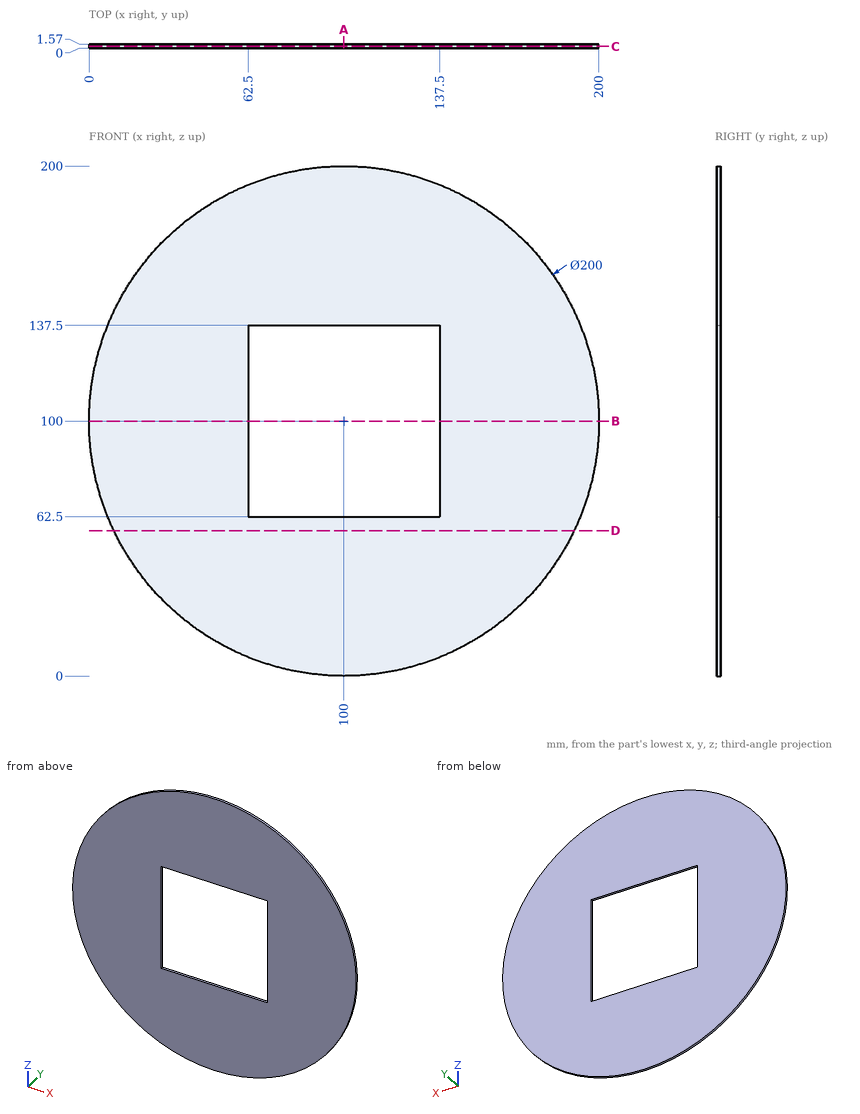
Here's the drawing with two shaded views (mm, measured from the low corner). I have some questions. Give positions to 0.01 mm unless a question says otherwise; leave off trailing zeros. Loops run counter-clockwise (first coordinate to the right, second up) from the corner with the lowest first, then second, coordinate; pieces in that order, holes last. Notation, with made-up numbers: (-14, 69) - (25, 69) arc R32 cw to (25, 97) - close; hole circle Ø7 at (62.25, 63). An arc over 180 degrees is marked (long way). Answer in a Markdown table with one row per item. Add a question column.
Q1. Please list where these lines run through material, in increasing order: L1, parallel to X at y = 0.9, z = 108; L2, parallel to X at y = 1, z = 130; L3, parallel to Z at x = 86.5, y = 0.85. Write a range as from..to.
Q2. If we section it at D-D (z = 57): List the corners of the cut face in (x, y) for me.
Q3. If we section it at B-B (z = 100): List the corners of the cut face in (x, y) for me, plus the area to 3 significant figures.
Q4. If we section it at A-A (x = 100): List the corners of the cut face in (y, z) for me.
Q5. For pin 1 (0.5 mm diameter, centred on y = 0.5, z = 88, fed in from +X); pin 2 (0.8 mm diameter, centred on x = 92, y = 1, fed in from -Z), each with a flat end and sliding along its axis, tell me the tip position at first contact or that it passes through.
Q6. If we section it at C-C (y = 0.6): List the corners of the cut face in (x, z) for me.
The answers:
| question | item | result |
|---|---|---|
| 1 | L1 | x = 0.32..62.5, 137.5..199.68 |
| 1 | L2 | x = 4.61..62.5, 137.5..195.39 |
| 1 | L3 | z = 0.92..62.5, 137.5..199.08 |
| 2 | outline | (9.72, 0) - (190.28, 0) - (190.28, 1.57) - (9.72, 1.57) - close |
| 3 | outline | (0, 0) - (62.5, 0) - (62.5, 1.57) - (0, 1.57) - close; (137.5, 0) - (200, 0) - (200, 1.57) - (137.5, 1.57) - close |
| 3 | area | 196 mm^2 |
| 4 | outline | (0, 0) - (1.57, 0) - (1.57, 62.5) - (0, 62.5) - close; (0, 137.5) - (1.57, 137.5) - (1.57, 200) - (0, 200) - close |
| 5 | pin 1 | stops at x = 199.31 |
| 5 | pin 2 | stops at z = 0.29 |
| 6 | outline | circle Ø200 at (100, 100); hole (62.5, 62.5) - (137.5, 62.5) - (137.5, 137.5) - (62.5, 137.5) - close |
